Autodesk Inventor part; units mm, degrees
ref_plane "Work Plane1" through (0, 0, 80) normal (0, 0, 1) x (1, 0, 0)
ref_plane "Work Plane2" through (0, 0, 0) normal (0, -1, 0) x (1, 0, 0)
ref_plane "Work Plane3" through (0, 0, 0) normal (0, 0, -1) x (-1, 0, 0)
sketch "Sketch1" plane through (0, 0, 0) normal (0, 0, 1) x (1, 0, 0)
  line L0 (0, 0) -> (130, 0)
  line L1 (130, 0) -> (193.6396, 63.6396)
  line L2 (0, 0) -> (-63.6396, 63.6396)
  arc A0 (193.6396, 63.6396) -> (-63.6396, 63.6396) centre (65, -144.7193) ccw
  dimension "d0" = 130
  dimension "d1" = 90
  dimension "d2" = 135
  dimension "d3" = 90
extrude "Extrusion1" add sketch "Sketch1" along normal blind 80
ref_plane "Work Plane1" through (0, 0, 80) normal (0, 0, 1) x (1, 0, 0)
sketch "Sketch2" plane through (0, 0, 80) normal (0, 0, 1) x (1, 0, 0)
  line L0 (-63.6396, 63.6396) -> (0, 0)
  line L1 (0, 0) -> (-42.4264, 42.4264)
  line L2 (0, 0) -> (130, 0)
  line L3 (0, 0) -> (130, 0)
  line L4 (130, 0) -> (172.4264, 42.4264)
  line L5 (130, 0) -> (193.6396, 63.6396)
  arc A0 (172.4264, 42.4264) -> (-42.4264, 42.4264) centre (65, -155.2225) ccw
  dimension "d7" = 60
  dimension "d8" = 60
extrude "Extrusion2" cut sketch "Sketch2" against normal blind 30
ref_plane "Work Plane2" through (0, 0, 0) normal (0, -1, 0) x (1, 0, 0)
sketch "Sketch4" plane through (0, 0, 0) normal (0, -1, 0) x (1, 0, 0)
  line L0 (-42.4264, 50) -> (-42.4264, 80)
  line L1 (-42.4264, 70) -> (172.4264, 70)
  line L2 (172.4264, 80) -> (172.4264, 50)
  line L3 (172.4264, 70) -> (172.4264, 80)
  line L4 (172.4264, 80) -> (-42.4264, 80)
  line L5 (193.6396, 80) -> (-63.6396, 80)
  line L6 (130, 50) -> (0, 50)
  point P0 (0, 0)
  dimension "d12" = 20
extrude "Extrusion3" add sketch "Sketch4" against normal blind 70
ref_plane "Work Plane3" through (0, 0, 0) normal (0, 0, -1) x (-1, 0, 0)
sketch "Sketch5" plane through (0, 0, 0) normal (0, 0, -1) x (-1, 0, 0)
  line L0 (-172.4264, 0) -> (-172.4264, 42.4264)
  line L1 (-172.4264, 42.4264) -> (-130, 0)
  line L2 (-172.4264, 0) -> (-172.4264, 42.4264)
  line L3 (-172.4264, 42.4264) -> (-130, 0)
  line L4 (42.4264, 0) -> (-172.4264, 0)
  line L5 (-130, 0) -> (-172.4264, 0)
  line L6 (-130, 0) -> (0, 0)
  line L7 (42.4264, 42.4264) -> (42.4264, 0)
  line L8 (63.6396, 63.6396) -> (0, 0)
  line L9 (42.4264, 42.4264) -> (0, 0)
  line L10 (0, 0) -> (42.4264, 0)
extrude "Extrusion4" cut sketch "Sketch5" against normal blind 80
ref_plane "Work Plane4" through (-63.6396, 63.6396, 80) normal (-0.7071, -0.7071, 0) x (-0.7071, 0.7071, 0)
sketch "Sketch6" plane through (-63.6396, 63.6396, 80) normal (-0.7071, -0.7071, 0) x (-0.7071, 0.7071, 0)
  circle A0 centre (-20.8328, 61.1519) radius 17
  circle A1 centre (-67.5207, 61.1519) radius 17
  point P0 (-90, 80)
  dimension "d19" = 34
  dimension "d21" = 34
extrude "Extrusion5" add sketch "Sketch6" along normal blind 15
sketch "Sketch7" plane through (-59.5152, 38.302, 18.8481) normal (-0.7071, -0.7071, 0) x (-0.7071, 0.7071, 0)
  circle A0 centre (0, 0) radius 12.5
  circle A1 centre (-46.6879, 0) radius 17
  circle A2 centre (-46.6879, 0) radius 12.5
  point P0 (-69.1672, 18.8481)
  dimension "d24" = 25
  dimension "d25" = 25
extrude "Extrusion6" cut sketch "Sketch7" against normal blind 20 contours A0
sketch "Sketch8" plane through (-26.5019, 5.2887, 18.8481) normal (-0.7071, -0.7071, 0) x (-0.7071, 0.7071, 0)
  circle A0 centre (0, 0) radius 12.5
  point P0 (-22.4793, 18.8481)
  dimension "d28" = 25
extrude "Extrusion7" cut sketch "Sketch8" against normal blind 20
properties part number "Calliper" material "Steel, Alloy"
Work out the finished part from the listing and answer in its coordinate system (mm). A direction names the side the tool comes from. Round coordinates to 2 decimals unless told otherwise and drop trailing zeros. Loops run counter-clockwise (first coordinate to the right, second up) from the corner with the lowest first, then second, coordinate; pieces in that order, holes last. Notation, with made-up numbers: (45, 75.5) - (74, 75.5) arc R24 cw to (74, 91.5) - close; hole circle Ø10 at (-18, 30.5). An arc over 180 degrees is marked (long way). Use one line per item in the form item = value. Start each with the question number.
(1) Consider line 1 (Z direction, x = 38, y = 59.5); line 2 (Z direction, x = -14, y = 1); line 3 (X direction, y = 20, z = 29). Determine where each line is inside the solid, lowest interval first.
(2) Find section D-D on z = 74. Determine the outline of the cut face in (x, y).
(3) Find section A-A on y = 22.5. Give the number of separate pieces and of enclosed holes in the cut face, and give its area (3 significant figures).
(4) Find section B-B on x = 40. Determine the outline of the cut face in (y, z), and give its area (3 significant figures).
(5) Flat-ended cylindrical pins translate along their axes: P1, Ø1, axis at y = 65, z = 64.5, coming from the +X side; P2, Ø4, axis at y = 63.5, z = 30, coming from the +X side; P3, Ø3, axis at x = 76, z = 74.5, coming from the -Y side. Find the tip coordinate at first contact, or state that the pin passes through.
(6) Determine the mould class of faces 6 (the face through (-27.96, 20.69, 15.09)), 7 (the face through (-59.459, 38.246, 6.176)), 8 (the face through (-65.6, 55.15, 23.95)), 9 (the face through (-45.528, 38.261, 26.454)) for opening direction Z: +Z half, -Z half, draft (parallel to the pull), parting line (faces both ways), or undercut.
(7) Find section C-C on y = 66.5. Determine the outline of the cut face in (x, z).
(8) Which of the six approach directions +Z, -Z, +X, -X, +Y, -Y give full straight-line access (tool end or side, diameter ignored) to faces 1 (the face through (-45.248, 52.322, 18.673)), 2 (the face through (63, 35, 50)), 3 (the face through (-26.446, 5.233, 6.176)), 4 (the face through (63, 51, 0)), 5 (the face through (64, 0, 25))?
Answer list:
q1.line_1 = 0 to 50, 70 to 80
q1.line_2 = 6.68 to 14.94, 22.76 to 31.02
q1.line_3 = -31.07 to -22.1, -12.93 to 150
q2.outline = (-63.64, 63.64) - (0, 0) - (130, 0) - (193.64, 63.64) arc R244.87 ccw to start
q3.separate_pieces = 2
q3.enclosed_holes = 1
q3.area = 10,500 mm^2
q4.outline = (0, 0) - (98.87, 0) - (98.87, 80) - (0, 80) - (0, 70) - (68.34, 70) - (68.34, 50) - (0, 50) - close
q4.area = 6,540 mm^2
q5.P1 = 192.24
q5.P2 = 193.64
q5.P3 = 0
q6.face_6 = undercut
q6.face_7 = draft
q6.face_8 = parting line
q6.face_9 = undercut
q7.outline = (-58.89, 0) - (188.89, 0) - (188.89, 80) - (-58.89, 80) - close; hole (26.99, 50) - (103.01, 50) - (103.01, 70) - (26.99, 70) - close
q8.face_1 = none
q8.face_2 = -Y
q8.face_3 = +Z, -Z, -X, -Y
q8.face_4 = -Z, +X, -X, +Y, -Y
q8.face_5 = +Z, -Z, +X, -Y
